from build123d import *

# Parameters (mm, degrees)
SKETCH1_W           = 184
SKETCH1_H           = 50
BOSS_EXTRUDE2_DEPTH = 6
SKETCH7_W           = 6
SKETCH7_H           = 6
CUT_EXTRUDE3_DEPTH  = 6
SKETCH8_W           = 50
SKETCH8_H           = 15
CUT_EXTRUDE4_DEPTH  = 6
SKETCH9_W           = 6
SKETCH9_H           = 6
BOSS_EXTRUDE3_DEPTH = 6


with BuildPart() as part:
    # Sketch1 → Boss-Extrude2 (new body)
    with BuildSketch(Plane.XY):
        with Locations((0, 25)):
            Rectangle(SKETCH1_W, SKETCH1_H)
    extrude(amount=BOSS_EXTRUDE2_DEPTH)

    # Sketch7 → Cut-Extrude3 (cut)
    with BuildSketch(Plane.XY):
        with Locations((77, 47)):
            Rectangle(SKETCH7_W, SKETCH7_H)
        with Locations((26, 47)):
            Rectangle(SKETCH7_W, SKETCH7_H)
        with Locations((-77, 47)):
            Rectangle(SKETCH7_W, SKETCH7_H)
        with Locations((-26, 47)):
            Rectangle(SKETCH7_W, SKETCH7_H)
    extrude(amount=CUT_EXTRUDE3_DEPTH, mode=Mode.SUBTRACT)

    # Sketch8 → Cut-Extrude4 (cut)
    with BuildSketch(Plane(origin=(0, 0, 0), x_dir=(-1, 0, 0), z_dir=(0, 0, -1))):
        with Locations((0, 32.5)):
            Rectangle(SKETCH8_W, SKETCH8_H)
    extrude(amount=-CUT_EXTRUDE4_DEPTH, mode=Mode.SUBTRACT)

    # Sketch9 → Boss-Extrude3 (add)
    with BuildSketch(Plane.XZ):
        with Locations((-83, 3)):
            Rectangle(SKETCH9_W, SKETCH9_H)
        with Locations((-33, 3)):
            Rectangle(SKETCH9_W, SKETCH9_H)
        with Locations((33, 3)):
            Rectangle(SKETCH9_W, SKETCH9_H)
        with Locations((83, 3)):
            Rectangle(SKETCH9_W, SKETCH9_H)
    extrude(amount=BOSS_EXTRUDE3_DEPTH)


solid = part.part
Work out the finished part from the listing and answer in its coordinate system (mm). A direction names the side the tool comes from. Give positions to 0.01 mm unless a question says otherwise; leave off trailing zeros. Order: outer loops, then holes, each group sorted by start corner. A loop starts at its lowest first (then second) coordinate and runs counter-clockwise, first axis right, second up. Notation, with made-up numbers: (-24.75, 12.25) - (13.25, 12.25) arc R7 ccw to (13.25, 21.25) - close; hole circle Ø2 at (32.5, 78.5). An arc over 180 degrees is marked (long way). Answer as CSV lines item,"result". Start each with the question number.
Q1. Given pin 1 Ø1.8 at (x, z) = (-88.5, 1.5) entering from -Y; pin 2 Ø1.8 at (y, z) = (-2.5, 3) entering from -X; pin 3 Ø1.8 at (y, z) = (-4.5, 4.5) entering from +X, each flat-ended and moving along its own axis, determine where each tip first touches the part or whether it passes through.
Q2. The part is cut by section C-C (x = -45.5). Write down the section's boundary in (y, z), then the cut area to 3 significant figures.
Q3. The part is cut by section B-B (x = -4.5). Write down the section's boundary in (y, z), then the cut area to 3 significant figures.
Q4. The part is cut by section A-A (y = 35.5). Write down the section's boundary in (x, z), then the cut area to 3 significant figures.
Q5. Find the intervals of material crossed by L1, parallel to X at y = 45, z = 2.45; L2, parallel to X at y = 39, z = 3.35; L3, parallel to Y at x = -20, z = 4.05, in increasing order. Write a range as [from, to].
Q6. The mould has two halves that part along Y. Classify faces 6 (the face through (23, 47, 3)), 7 (the face through (0, 25, 3)), 8 (the face through (-26, 44, 3)): +Y half, -Y half, draft (parallel to the pull), parting line (faces both ways), or undercut.
Q7. For faces 1 (the face through (-25, 32, 3)), 2 (the face through (26, 44, 3)), 3 (the face through (-52, 50, 3)), 4 (the face through (-86, -3, 3)), 5 (the face through (36, -3, 3)), determine the directions among +Z, -Z, +X, -X, +Y, -Y from which every point of the face is accessible in a straight line to the end or side of a thin tool.
Check result:
1,pin 1,"stops at y = 0"
1,pin 2,"stops at x = -86"
1,pin 3,"stops at x = 86"
2,outline,"(0, 0) - (50, 0) - (50, 6) - (0, 6) - close"
2,area,"300 mm²"
3,outline,"(0, 0) - (25, 0) - (25, 6) - (0, 6) - close; (40, 0) - (50, 0) - (50, 6) - (40, 6) - close"
3,area,"210 mm²"
4,outline,"(-92, 0) - (-25, 0) - (-25, 6) - (-92, 6) - close; (25, 0) - (92, 0) - (92, 6) - (25, 6) - close"
4,area,"804 mm²"
5,L1,"x = [-92, -80], [-74, -29], [-23, 23], [29, 74], [80, 92]"
5,L2,"x = [-92, -25], [25, 92]"
5,L3,"y = [0, 25], [40, 50]"
6,face 6,"draft"
6,face 7,"undercut"
6,face 8,"+Y half"
7,face 1,"+Z, -Z"
7,face 2,"+Z, -Z, +Y"
7,face 3,"+Z, -Z, +X, -X, +Y"
7,face 4,"+Z, -Z, -X, -Y"
7,face 5,"+Z, -Z, -Y"
